from build123d import *

# Parameters (mm, degrees)
F0_R     = 152.4
F0_R_2   = 76.2
F0_R_3   = 12.7
F1_DEPTH = 63.5
F3_DEPTH = 63.5


with BuildPart() as f1:
    # F0 (on Front) → F1 (new body, symmetric)
    with BuildSketch(Plane.XZ):
        Circle(F0_R)
        Circle(F0_R_2, mode=Mode.SUBTRACT)
        Circle(F0_R_2)
        Circle(F0_R_3, mode=Mode.SUBTRACT)
    extrude(amount=F1_DEPTH, both=True)

    # F2 (on Front) → F3 (cut, symmetric)
    with BuildSketch(Plane.XZ):
        with BuildLine():
            ThreePointArc((-18.8071139829, 138.4282574608), (0, 139.7), (18.8071139829, 138.4282574608))
            Line((18.8071139829, 138.4282574608), (23.2434776929, 150.6170665786))
            ThreePointArc((23.2434776929, 150.6170665786), (0, 152.4), (-23.2434776929, 150.6170665786))
            Line((-23.2434776929, 150.6170665786), (-18.8071139829, 138.4282574608))
        make_face()
        with BuildLine():
            ThreePointArc((-60.6633123632, 125.8413784616), (-43.1696741142, 132.8625953264), (-24.890055751, 137.4648141333))
            Line((-24.890055751, 137.4648141333), (-24.4373722945, 150.4279722503))
            ThreePointArc((-24.4373722945, 150.4279722503), (-47.0941899427, 144.9410130834), (-68.6490941369, 136.0627130194))
            Line((-68.6490941369, 136.0627130194), (-60.6633123632, 125.8413784616))
        make_face()
        with BuildLine():
            ThreePointArc((-96.5813630633, 100.9362685502), (-82.1135997453, 113.0196741142), (-66.1508134087, 123.0453570248))
            Line((-66.1508134087, 123.0453570248), (-69.7261220165, 135.5139399049))
            ThreePointArc((-69.7261220165, 135.5139399049), (-89.5784724494, 123.2941899427), (-107.3348589404, 108.1895931051))
            Line((-107.3348589404, 108.1895931051), (-96.5813630633, 100.9362685502))
        make_face()
        with BuildLine():
            ThreePointArc((-123.0453570248, 66.1508134087), (-113.0196741142, 82.1135997453), (-100.9362685502, 96.5813630633))
            Line((-100.9362685502, 96.5813630633), (-108.1895931051, 107.3348589404))
            ThreePointArc((-108.1895931051, 107.3348589404), (-123.2941899427, 89.5784724494), (-135.5139399049, 69.7261220165))
            Line((-135.5139399049, 69.7261220165), (-123.0453570248, 66.1508134087))
        make_face()
        with BuildLine():
            ThreePointArc((-137.4648141333, 24.890055751), (-132.8625953264, 43.1696741142), (-125.8413784616, 60.6633123632))
            Line((-125.8413784616, 60.6633123632), (-136.0627130194, 68.6490941369))
            ThreePointArc((-136.0627130194, 68.6490941369), (-144.9410130834, 47.0941899427), (-150.4279722503, 24.4373722945))
            Line((-150.4279722503, 24.4373722945), (-137.4648141333, 24.890055751))
        make_face()
        with BuildLine():
            ThreePointArc((-138.4282574608, -18.8071139829), (-139.7, 0), (-138.4282574608, 18.8071139829))
            Line((-138.4282574608, 18.8071139829), (-150.6170665786, 23.2434776929))
            ThreePointArc((-150.6170665786, 23.2434776929), (-152.4, 0), (-150.6170665786, -23.2434776929))
            Line((-150.6170665786, -23.2434776929), (-138.4282574608, -18.8071139829))
        make_face()
        with BuildLine():
            ThreePointArc((-125.8413784616, -60.6633123632), (-132.8625953264, -43.1696741142), (-137.4648141333, -24.890055751))
            Line((-137.4648141333, -24.890055751), (-150.4279722503, -24.4373722945))
            ThreePointArc((-150.4279722503, -24.4373722945), (-144.9410130834, -47.0941899427), (-136.0627130194, -68.6490941369))
            Line((-136.0627130194, -68.6490941369), (-125.8413784616, -60.6633123632))
        make_face()
        with BuildLine():
            ThreePointArc((-100.9362685502, -96.5813630633), (-113.0196741142, -82.1135997453), (-123.0453570248, -66.1508134087))
            Line((-123.0453570248, -66.1508134087), (-135.5139399049, -69.7261220165))
            ThreePointArc((-135.5139399049, -69.7261220165), (-123.2941899427, -89.5784724494), (-108.1895931051, -107.3348589404))
            Line((-108.1895931051, -107.3348589404), (-100.9362685502, -96.5813630633))
        make_face()
        with BuildLine():
            ThreePointArc((-66.1508134087, -123.0453570248), (-82.1135997453, -113.0196741142), (-96.5813630633, -100.9362685502))
            Line((-96.5813630633, -100.9362685502), (-107.3348589404, -108.1895931051))
            ThreePointArc((-107.3348589404, -108.1895931051), (-89.5784724494, -123.2941899427), (-69.7261220165, -135.5139399049))
            Line((-69.7261220165, -135.5139399049), (-66.1508134087, -123.0453570248))
        make_face()
        with BuildLine():
            ThreePointArc((-24.890055751, -137.4648141333), (-43.1696741142, -132.8625953264), (-60.6633123632, -125.8413784616))
            Line((-60.6633123632, -125.8413784616), (-68.6490941369, -136.0627130194))
            ThreePointArc((-68.6490941369, -136.0627130194), (-47.0941899427, -144.9410130834), (-24.4373722945, -150.4279722503))
            Line((-24.4373722945, -150.4279722503), (-24.890055751, -137.4648141333))
        make_face()
        with BuildLine():
            ThreePointArc((18.8071139829, -138.4282574608), (0, -139.7), (-18.8071139829, -138.4282574608))
            Line((-18.8071139829, -138.4282574608), (-23.2434776929, -150.6170665786))
            ThreePointArc((-23.2434776929, -150.6170665786), (0, -152.4), (23.2434776929, -150.6170665786))
            Line((23.2434776929, -150.6170665786), (18.8071139829, -138.4282574608))
        make_face()
        with BuildLine():
            ThreePointArc((60.6633123632, -125.8413784616), (43.1696741142, -132.8625953264), (24.890055751, -137.4648141333))
            Line((24.890055751, -137.4648141333), (24.4373722945, -150.4279722503))
            ThreePointArc((24.4373722945, -150.4279722503), (47.0941899427, -144.9410130834), (68.6490941369, -136.0627130194))
            Line((68.6490941369, -136.0627130194), (60.6633123632, -125.8413784616))
        make_face()
        with BuildLine():
            ThreePointArc((96.5813630633, -100.9362685502), (82.1135997453, -113.0196741142), (66.1508134087, -123.0453570248))
            Line((66.1508134087, -123.0453570248), (69.7261220165, -135.5139399049))
            ThreePointArc((69.7261220165, -135.5139399049), (89.5784724494, -123.2941899427), (107.3348589404, -108.1895931051))
            Line((107.3348589404, -108.1895931051), (96.5813630633, -100.9362685502))
        make_face()
        with BuildLine():
            ThreePointArc((123.0453570248, -66.1508134087), (113.0196741142, -82.1135997453), (100.9362685502, -96.5813630633))
            Line((100.9362685502, -96.5813630633), (108.1895931051, -107.3348589404))
            ThreePointArc((108.1895931051, -107.3348589404), (123.2941899427, -89.5784724494), (135.5139399049, -69.7261220165))
            Line((135.5139399049, -69.7261220165), (123.0453570248, -66.1508134087))
        make_face()
        with BuildLine():
            ThreePointArc((137.4648141333, -24.890055751), (132.8625953264, -43.1696741142), (125.8413784616, -60.6633123632))
            Line((125.8413784616, -60.6633123632), (136.0627130194, -68.6490941369))
            ThreePointArc((136.0627130194, -68.6490941369), (144.9410130834, -47.0941899427), (150.4279722503, -24.4373722945))
            Line((150.4279722503, -24.4373722945), (137.4648141333, -24.890055751))
        make_face()
        with BuildLine():
            ThreePointArc((138.4282574608, 18.8071139829), (139.7, 0), (138.4282574608, -18.8071139829))
            Line((138.4282574608, -18.8071139829), (150.6170665786, -23.2434776929))
            ThreePointArc((150.6170665786, -23.2434776929), (152.4, 0), (150.6170665786, 23.2434776929))
            Line((150.6170665786, 23.2434776929), (138.4282574608, 18.8071139829))
        make_face()
        with BuildLine():
            ThreePointArc((125.8413784616, 60.6633123632), (132.8625953264, 43.1696741142), (137.4648141333, 24.890055751))
            Line((137.4648141333, 24.890055751), (150.4279722503, 24.4373722945))
            ThreePointArc((150.4279722503, 24.4373722945), (144.9410130834, 47.0941899427), (136.0627130194, 68.6490941369))
            Line((136.0627130194, 68.6490941369), (125.8413784616, 60.6633123632))
        make_face()
        with BuildLine():
            ThreePointArc((100.9362685502, 96.5813630633), (113.0196741142, 82.1135997453), (123.0453570248, 66.1508134087))
            Line((123.0453570248, 66.1508134087), (135.5139399049, 69.7261220165))
            ThreePointArc((135.5139399049, 69.7261220165), (123.2941899427, 89.5784724494), (108.1895931051, 107.3348589404))
            Line((108.1895931051, 107.3348589404), (100.9362685502, 96.5813630633))
        make_face()
        with BuildLine():
            ThreePointArc((66.1508134087, 123.0453570248), (82.1135997453, 113.0196741142), (96.5813630633, 100.9362685502))
            Line((96.5813630633, 100.9362685502), (107.3348589404, 108.1895931051))
            ThreePointArc((107.3348589404, 108.1895931051), (89.5784724494, 123.2941899427), (69.7261220165, 135.5139399049))
            Line((69.7261220165, 135.5139399049), (66.1508134087, 123.0453570248))
        make_face()
        with BuildLine():
            ThreePointArc((24.890055751, 137.4648141333), (43.1696741142, 132.8625953264), (60.6633123632, 125.8413784616))
            Line((60.6633123632, 125.8413784616), (68.6490941369, 136.0627130194))
            ThreePointArc((68.6490941369, 136.0627130194), (47.0941899427, 144.9410130834), (24.4373722945, 150.4279722503))
            Line((24.4373722945, 150.4279722503), (24.890055751, 137.4648141333))
        make_face()
    extrude(amount=F3_DEPTH, both=True, mode=Mode.SUBTRACT)


solid = f1.part
Check sheet for the modelled part. Datum: model origin and axes. Units: mm. A direction names the side the tool comes from. Give positions to 0.01 mm unless a question says otherwise; leave off trailing zeros. Loops run counter-clockwise (first coordinate to the right, second up) from the corner with the lowest first, then second, coordinate; pieces in that order, holes last. Notation, with made-up numbers: M 31,49 L 59,49 A17 ccw 59,62 Z; hole C 29.25,-17 d5. An arc over 180 degrees is marked long. Answer as a JSON object with one key per item and string values. Group by question number.
Q1. Cross-section at D-D on z = 45. Record the cut outline in (x, y), then the cut area to 3 significant figures.
Q2. Cross-section at A-A on x = 0. Record the cut outline in (y, z), then the cut area to 3 significant figures.
Q3. Cross-section at C-C on x = 90.5. Record the cut outline in (y, z).
Q4. Material ranges on line 1 along X through (y, z) = (-20, -130); line 2 along X through (y, z) = (0.5, -101); line 3 along Z through (x, y) = (-106, -17.5) (3 decimals), recorded low to high. Write a range as [from, to].
Q5. Release check for a two-part mould opening along X. For faces 6 (the flat face through (67.963, 0.889, 129.367)), 7 (the flat face through (-144.437, 0.889, 20.994)), 8 (the cylindrical face through (43.42, 0.89, -132.78)) record: released by +X, released by -X, zero draft, split by the parting line, or undercut.
Q6. Go/stop test with flat-tipped pins: P1, Ø12, axis at x = 78, y = -27, coming from the -Z side; P2, Ø1.5, axis at y = -13, z = 117, coming from the +X side; P3, Ø10, axis at x = -65, y = -4.5, coming from the -Z side. Record where each tip stops, or that it passes through.
Q7. Cross-section at B-B on z = 0. Record the cut outline in (x, y), then the cut area to 3 significant figures.
Q8. Access from +Z, -Z, +X, -X, +Y, -Y to the whole of each face (thin tool, end or side, straight path). Record for faces 1 (the cylindrical face through (132.78, 0.89, 43.42)), 2 (the flat face through (64.6, -0.89, 130.88)), 3 (the cylindrical face through (-2.75, 0.89, -12.4)), 4 (the flat face through (-67.913, 0.889, 129.192)), 5 (the flat face through (21.056, 0.889, -144.608)).
Evaluation:
{
 "1": {"outline": "M -132.25,-63.5 L 132.25,-63.5 L 132.25,63.5 L -132.25,63.5 Z", "area": "33,600 mm2"},
 "2": {"outline": "M -63.5,-139.7 L 63.5,-139.7 L 63.5,-12.7 L -63.5,-12.7 Z; M -63.5,12.7 L 63.5,12.7 L 63.5,139.7 L -63.5,139.7 Z", "area": "32,300 mm2"},
 "3": {"outline": "M -63.5,-106.42 L 63.5,-106.42 L 63.5,106.42 L -63.5,106.42 Z"},
 "4": {"line 1": "x = [-68.15, -63.91], [-51.15, 51.15], [63.91, 68.15]", "line 2": "x = [-103.92, -96.68], [-96.51, 96.51], [96.68, 103.92]", "line 3": "z = [-107.289, -104.089], [-90.995, 90.995], [104.089, 107.289]"},
 "5": {"face 6": "released by +X", "face 7": "released by -X", "face 8": "undercut"},
 "6": {"P1": "stops at z = -119.72", "P2": "stops at x = 77.47", "P3": "stops at z = -136.06"},
 "7": {"outline": "M -139.7,-63.5 L -12.7,-63.5 L -12.7,63.5 L -139.7,63.5 Z; M 12.7,-63.5 L 139.7,-63.5 L 139.7,63.5 L 12.7,63.5 Z", "area": "32,300 mm2"},
 "8": {"face 1": "+X, +Y, -Y", "face 2": "+Z, +Y, -Y", "face 3": "+Y, -Y", "face 4": "-X, +Y, -Y", "face 5": "-Z, +Y, -Y"}
}
